Geometry: final body of the model. Coordinates: model frame, mm. A direction names the side the tool comes from. Give positions to 0.01 mm unless a question says otherwise; leave off trailing zeros. Loops run counter-clockwise (first coordinate to the right, second up) from the corner with the lowest first, then second, coordinate; pieces in that order, holes last. Notation, with made-up numbers: (71.25, 32.25) -> (125.25, 32.25) arc R30 cw to (125.25, 69.25) -> close; hole circle Ø11 at (41, 78.25). An arc over 180 degrees is marked (long way). Answer in a Markdown table with one row per item. Add a question column.
1) Section query C-C (y = -56.5). Give the number of separate pieces and of enclosed holes in the cut face, plus the area to 3 significant figures.
2) Access query for faces 1 (the cylindrical face through (-103.3, -79.21, 0.09)), 2 (the cylindrical face through (-22.713, -102.283, 42.351)). Directions: +Z, -Z, +X, -X, +Y, -Y. A direction counts if a zero-diameter tool reaches every point of the face in a straight line with its end or side. Return the directions, or none.
3) Draft query along X for faces 3 (the flat face through (1, 1, 6.35)), 4 (the cylindrical face through (93.88, 29.56, 43.92)), 5 (the flat face through (-87.4, 58.5, 6.35)), 6 (the conical face through (97.055, 30.564, 82.396)). Return one class per face: +X half, -X half, draft (parallel to the pull), parting line (faces both ways), or undercut.
4) Section query A-A (y = 0). Return the cut outline in (x, z) (3 decimals).
5) First-contact query: P1, Ø3, axis at x = -53, y = -65, coming from the +Z side; P2, Ø15.5, axis at x = 0, y = -117.475, coming from the +Z side; P3, Ø17.5, axis at x = -117.475, y = 0, coming from the -Z side; P4, Ø2, axis at y = 28, z = 61, coming from the +X side. Flat tips, straight axial feed; report the tip coordinate or a pass-through.
6) Section query B-B (z = 69.5). Return the cut outline in (x, y) (3 decimals).
7) Line query: line 1 (Y direction, x = 1.5, z = -0.5); line 2 (Z direction, x = -86.5, y = 18); line 3 (Y direction, x = 69, z = 58.5). Output: solid intervals per line, ascending. Write a range as from..to.
```python
from build123d import *

# Parameters (mm, degrees)
SKETCH1_R                     = 130.175
SKETCH1_R_2                   = 104.775
BOSS_EXTRUDE1_DEPTH           = 6.35
SKETCH2_R                     = 104.775
SKETCH2_R_2                   = 98.425
BOSS_EXTRUDE2_DEPTH           = 82.55
SKETCH3_R                     = 98.425
BOSS_EXTRUDE3_DEPTH           = 6.35
CHAMFER1_SIZE                 = 3.175
F_1_2_CLEARANCE_HOLE1_D       = 13.49248
CIRPATTERN1_COUNT             = 12
MOVE_FACE1_BY                 = 6.35
TAP_DRILL_FOR_6_32_TAP1_D     = 2.7051
TAP_DRILL_FOR_6_32_TAP1_DEPTH = 6.35
TAP_DRILL_FOR_6_32_TAP1_TIP   = 0.81269403


with BuildPart() as part:
    # Sketch1 → Boss-Extrude1 (new body)
    with BuildSketch(Plane.XY):
        Circle(SKETCH1_R)
        Circle(SKETCH1_R_2, mode=Mode.SUBTRACT)
    extrude(amount=BOSS_EXTRUDE1_DEPTH)

    # Sketch2 → Boss-Extrude2 (add)
    with BuildSketch(Plane.XY):
        Circle(SKETCH2_R)
        Circle(SKETCH2_R_2, mode=Mode.SUBTRACT)
    extrude(amount=BOSS_EXTRUDE2_DEPTH)

    # Sketch3 → Boss-Extrude3 (add)
    with BuildSketch(Plane(origin=(0, 0, 0), x_dir=(-1, 0, 0), z_dir=(0, 0, -1))):
        Circle(SKETCH3_R)
    extrude(amount=-BOSS_EXTRUDE3_DEPTH)

    # Chamfer1
    chamfer1_edges = [part.edges().sort_by_distance(p)[0] for p in [
        (-104.775, 0, 82.55),
    ]]
    chamfer(chamfer1_edges, length=CHAMFER1_SIZE)

    # 1/2 Clearance Hole1 (through all)
    with Locations(Plane.XY.offset(6.35)):
        with Locations((0, 117.475)):
            f_1_2_clearance_hole1 = Hole(F_1_2_CLEARANCE_HOLE1_D / 2)

    # CirPattern1: 1/2 Clearance Hole1 ×12 about axis
    cirpattern1_axis = Axis((0, 0, 0), (0, 0, 1))
    for i in range(1, CIRPATTERN1_COUNT):
        add(f_1_2_clearance_hole1.rotate(cirpattern1_axis, i * 360 / CIRPATTERN1_COUNT), mode=Mode.SUBTRACT)

    # Move Face1: a face moved outward by 6.35
    extrude(part.faces().sort_by_distance((0, 0, 0))[0], amount=MOVE_FACE1_BY, dir=(0, 0, -1))

    # Tap Drill for #6-32 Tap1
    with Locations(Plane(origin=(-50.165, 20.32, 6.35), x_dir=(1, 0, 0), z_dir=(0, 0, 1))):
        with Locations((0, 0), (0, -40.64), (100.33, -52.07), (100.33, 11.43)):
            Hole(TAP_DRILL_FOR_6_32_TAP1_D / 2, depth=TAP_DRILL_FOR_6_32_TAP1_DEPTH)
            with Locations((0, 0, -(TAP_DRILL_FOR_6_32_TAP1_DEPTH + TAP_DRILL_FOR_6_32_TAP1_TIP / 2))):  # 118° drill point
                Cone(0, TAP_DRILL_FOR_6_32_TAP1_D / 2, TAP_DRILL_FOR_6_32_TAP1_TIP, mode=Mode.SUBTRACT)


solid = part.part
```
Evaluation:
| question | item | result |
|---|---|---|
| 1 | separate pieces | 3 |
| 1 | enclosed holes | 0 |
| 1 | area | 3,810 mm² |
| 2 | face 1 | +Z, -Z |
| 2 | face 2 | +Z |
| 3 | face 3 | undercut |
| 3 | face 4 | undercut |
| 3 | face 5 | draft |
| 3 | face 6 | parting line |
| 4 | outline | (-130.175, -6.35) -> (-124.221, -6.35) -> (-124.221, 6.35) -> (-130.175, 6.35) -> close; (-110.729, -6.35) -> (110.729, -6.35) -> (110.729, 6.35) -> (104.775, 6.35) -> (104.775, 79.375) -> (101.6, 82.55) -> (98.425, 82.55) -> (98.425, 6.35) -> (-98.425, 6.35) -> (-98.425, 82.55) -> (-101.6, 82.55) -> (-104.775, 79.375) -> (-104.775, 6.35) -> (-110.729, 6.35) -> close; (124.221, -6.35) -> (130.175, -6.35) -> (130.175, 6.35) -> (124.221, 6.35) -> close |
| 5 | P1 | z = 6.35 |
| 5 | P2 | z = 6.35 |
| 5 | P3 | z = -6.35 |
| 5 | P4 | x = 101.24 |
| 6 | outline | circle Ø209.55 at (0, 0); hole circle Ø196.85 at (0, 0) |
| 7 | line 1 | -130.17..-124.05, -110.9..110.9, 124.05..130.17 |
| 7 | line 2 | -6.35..6.35 |
| 7 | line 3 | -78.85..-70.19, 70.19..78.85 |
